The listing builds one solid part. Answer for the finished solid, in the listing's coordinates (mm). A direction names the side the tool comes from. Round coordinates to 2 decimals unless told otherwise and drop trailing zeros. Write each loop counter-clockwise with the first axis right and the second up, starting at its lowest first coordinate (ties: lowest second). Pieces come first, ordered by that corner, then holes. Notation, with made-up numbers: (3, 23.25) - (57, 23.25) arc R23 cw to (57, 42.25) - close; hole circle Ø1 at (17.25, 4). An arc over 180 degrees is marked (long way). Answer as CSV lines item,"result". Start each with the question number.
Item 1: Straight lines are drawn through the part: line 1 along X through (y, z) = (-3.25, 4.5); line 2 along Y through (x, z) = (4, 3.5); line 3 along Y through (x, z) = (4.5, 3.5). For each, find the intervals that lie inside material, in ascending order. Write a range as [from, to].
Item 2: A cutting plane is placed at A-A on z = 2. Determine the outline of the cut face in (x, y), and give its area (3 significant figures).
Item 3: For a pull along Y with two mould halves and no side action, classify faces 1 (the cylindrical face through (9.443, -2.974, 3.563)), 2 (the flat face through (-6, 2, -2)), 3 (the flat face through (0, 0, 0)), 4 (the conical face through (-1.12, -8.52, 5.79)) as pulls with the +Y half, pulls with the -Y half, needs draft (parallel to the pull), parting line crosses it, or undercut.
Item 4: A cutting plane is placed at B-B on z = 6.75. Determine the outline of the cut face in (x, y) (3 decimals).
Item 5: Which of the six approach directions +Z, -Z, +X, -X, +Y, -Y give full straight-line access (tool end or side, diameter ignored) to faces 5 (the conical face through (1.9, 3.65, -0.12)), 6 (the flat face through (0, 0, 3.3))?
Item 6: Flat-ended cylindrical pins translate along their axes: pin 1 (4 mm diameter, centred on x = -1.5, y = 1.5, fed in from -Z); pin 2 (1 mm diameter, centred on x = -0.5, y = -0.5, fed in from +Z); pin 3 (3 mm diameter, centred on x = -4.5, y = -1.5, fed in from -Z); pin 4 (4 mm diameter, centred on y = 4.5, z = 3.5, fed in from -X). Find the tip coordinate at first contact, or state that the pin passes through.
```python
from build123d import *

# Parameters (mm, degrees)
CHAMFER_1_SIZE      = 1
FILLET_1_R          = 0.4
SKETCH_2_R          = 1.5
CUT_EXTRUDE_1_DEPTH = 6.7
CHAMFER_2_SIZE      = 0.2
CHAMFER_2_SIZE_2    = 0.196243157


with BuildPart() as part:
    # 스케치1 → 회전1 (revolve)
    with BuildSketch(Plane(origin=(0, 0, 0), x_dir=(1, 0, 0), z_dir=(0, 1, 0))):
        with BuildLine():
            Line((0, 0), (4, 0))
            Line((4, 0), (5.894700278586023, 2))
            Line((5.894700278586023, 2), (9.9, 2))
            Line((9.9, 2), (9.900000000000002, -9))
            Line((9.900000000000002, -9), (8.700000000000008, -9))
            Line((8.700000000000008, -9), (8.5, -2.999999999999999))
            ThreePointArc((8.5, -2.999999999999999), (4.254277259758997, -3.290891769878769), (0, -3.4000000000000004))
            Line((0, -3.4000000000000004), (0, -3))
            Line((0, -3), (0, 0))
        make_face()
    revolve(axis=Axis((0, 0, 3), (0, 0, -1)))

    # 모따기1
    chamfer_1_edges = [part.edges().sort_by_distance(p)[0] for p in [
        (-9.900000000000002, -1.21e-15, 9),
        (-9.9, -1.21e-15, -2),
    ]]
    chamfer(chamfer_1_edges, length=CHAMFER_1_SIZE)

    # 필렛1
    # the kernel refuses this fillet: 0.4 mm, written as the material it takes off along each edge
    with BuildSketch(Plane(origin=(0, 0, 9), x_dir=(1, 0, 0), z_dir=(0, 1, 0))) as fillet_1_piece_1:
        with BuildLine():
            CenterArc((9.088461478811075, 0.35282045151089214), FILLET_1_R, 181.90915243299636, 59.981635971248124)
            Line((8.688683516019413, 0.3394945194178369), (8.68068795676358, 0.33922800077597515))
            Line((8.68068795676358, 0.33922800077597515), (8.692004440744174, -0.00026651864186178))
            Line((8.692004440744174, -0.00026651864186178), (8.700000000000008, -0.00799999999999912))
            ThreePointArc((8.700000000000008, -0.00799999999999912), (8.800000000000006, -0.00799999999999912), (8.896230770423783, -0.00705640903021099))
            Line((8.896230770423783, -0.00705640903021099), (8.900000000000004, 7.11e-15))
        make_face()
    revolve(axis=Axis((0, 0, 9), (0, 0, -1)), mode=Mode.SUBTRACT)
    with BuildSketch(Plane(origin=(0, 0, -2), x_dir=(1, 0, 0), z_dir=(0, 1, 0))) as fillet_1_piece_2:
        with BuildLine():
            CenterArc((5.894700278586023 + FILLET_1_R * 0.430137532673, -FILLET_1_R), FILLET_1_R, 90, 46.54870972712371)
            Line((5.894700278586023 - FILLET_1_R * 0.295821777418, -FILLET_1_R * 0.312262346464), (5.894700278586023 - FILLET_1_R * 0.31034096362, -FILLET_1_R * 0.298507593393))
            Line((5.894700278586023 - FILLET_1_R * 0.31034096362, -FILLET_1_R * 0.298507593393), (5.894700278586023 - FILLET_1_R * 0.00860275065346, FILLET_1_R * 0.02))
            Line((5.894700278586023 - FILLET_1_R * 0.00860275065346, FILLET_1_R * 0.02), (5.894700278586023 + FILLET_1_R * 0.430137532673, FILLET_1_R * 0.02))
            Line((5.894700278586023 + FILLET_1_R * 0.430137532673, FILLET_1_R * 0.02), (5.894700278586023 + FILLET_1_R * 0.430137532673, 0))
        make_face()
    revolve(axis=Axis((0, 0, -2), (0, 0, -1)), mode=Mode.SUBTRACT)

    # 스케치2 → 컷-돌출1 (cut)
    with BuildSketch(Plane.XY.offset(10)):
        Circle(SKETCH_2_R)
    extrude(amount=-CUT_EXTRUDE_1_DEPTH, mode=Mode.SUBTRACT)

    # 모따기2
    # the kernel refuses this chamfer: 0.2, 0.196243157 mm, written as the material it takes off along each edge
    with BuildSketch(Plane(origin=(6.4671513e-10, -1.09559634e-09, 3.3823067338827144), x_dir=(1.0, 7.303978568468729e-10, 0), z_dir=(7.303978568468729e-10, -1.0, 0))) as chamfer_2_piece_1_section:
        with BuildLine():
            Line((1.4999999993532855 + CHAMFER_2_SIZE * 0.999793216119, -CHAMFER_2_SIZE * 0.0203353141858), (1.4999999993532855 + CHAMFER_2_SIZE_2 * 6.59095382194e-09, -CHAMFER_2_SIZE_2 * 1.00000000151))
            Line((1.4999999993532855 + CHAMFER_2_SIZE_2 * 6.59095382194e-09, -CHAMFER_2_SIZE_2 * 1.00000000151), (1.4999999993532855, 0))
            ThreePointArc((1.4999999993532855, 0), (1.6028067115105318, -0.00204082683161744), (1.4999999993532855 + CHAMFER_2_SIZE * 0.999793216119, -CHAMFER_2_SIZE * 0.0203353141858))
        make_face()
    chamfer_2_piece_1 = revolve(axis=Axis((6.4671513e-10, -1.09559634e-09, 3.3823067338827144), (0, 0, 1)), mode=Mode.PRIVATE)
    chamfer_2_piece_1 = split(chamfer_2_piece_1, bisect_by=Plane(origin=(6.4671513e-10, -1.09559634e-09, 3.3), z_dir=(0, 0, 1)), keep=Keep.TOP, mode=Mode.PRIVATE)
    add(chamfer_2_piece_1, mode=Mode.SUBTRACT)


solid = part.part
```
Geometry says:
1,line 1,"x = [-9.35, -7.91], [7.91, 9.35]"
1,line 2,"y = [-9.06, -7.52], [7.52, 9.06]"
1,line 3,"y = [-8.82, -7.23], [7.23, 8.82]"
2,outline,"circle Ø19.8 at (0, 0)"
2,area,"308 mm^2"
3,face 1,"parting line crosses it"
3,face 2,"needs draft"
3,face 3,"undercut"
3,face 4,"undercut"
4,outline,"circle Ø19.8 at (0, 0); hole circle Ø17.25 at (0, 0)"
5,face 5,"-Z"
5,face 6,"+Z"
6,pin 1,"stops at z = -0.13"
6,pin 2,"stops at z = 3.3"
6,pin 3,"stops at z = -2"
6,pin 4,"stops at x = -9.58"
